Geometry: see drawing. Coordinates: mm, zero at the bounding-box minimum. Give positions to 0.01 mm unless a question says otherwise; leave off trailing zeros. Order: outer loops, then holes, each group sorted by start corner. A loop starts at its lowest first (then second) coordinate and runs counter-clockwise, first axis right, second up. Notation, with made-up numbers: (89.5, 10) -> (111.5, 10) arc R25 ccw to (111.5, 40) -> close; hole circle Ø5 at (79, 44). An arc over 180 degrees is marked (long way). One line per item, written item: value. Start each with the question number.
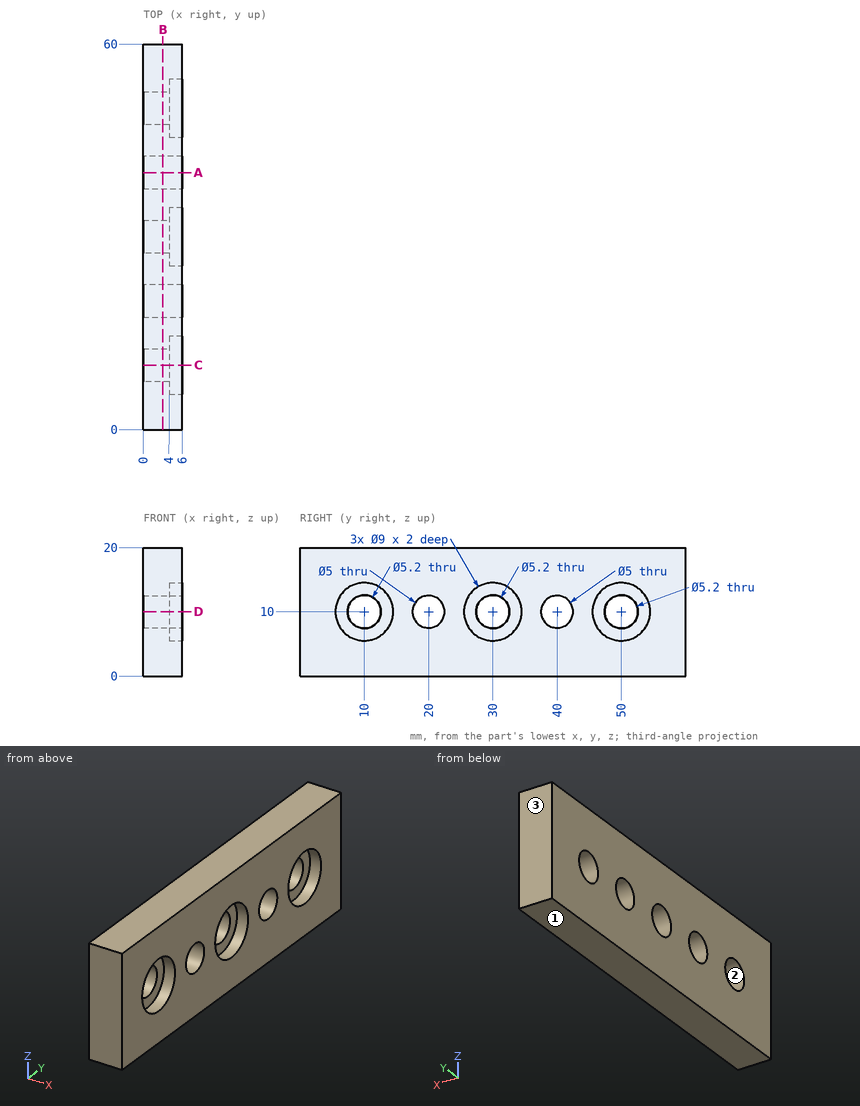
1. Pin query (flat end, axial travel): P1, Ø7, axis at y = 10, z = 10, coming from the +X side. Return the tip coordinate at first contact, or that it passes through.
2. Cut plane A-A, the plane y = 40. Return loops of the section in (x, z), then the cut area to 3 significant figures.
3. Draft query along Z for the marked faces 1, 2 and 3. Return one class per face: pulls with the +Z half, pulls with the -Z half, needs draft (parallel to the pull), parting line crosses it, or undercut.
4. Cut plane D-D, the plane z = 10. State how many separate pieces and enclosed holes the cut face has, then the cut area to 3 significant figures.
5. Cut plane B-B, the plane x = 3. Return loops of the section in (y, z).
6. Material intervals for L1, parallel to Z at x = 1.4, y = 10; L2, parallel to Z at x = 5.2, y = 50; L3, parallel to Y at x = 2, z = 12.25, sorted ascending. Write a range as [from, to].
7. Cut plane C-C, the plane y = 10. Return loops of the section in (x, z).
Answers follow:
1. P1: stops at x = 4
2. outline: (0, 0) -> (6, 0) -> (6, 7.5) -> (0, 7.5) -> close; (0, 12.5) -> (6, 12.5) -> (6, 20) -> (0, 20) -> close
2. area: 90.0 mm²
3. face 1: pulls with the -Z half
3. face 2: undercut
3. face 3: needs draft
4. separate pieces: 6
4. enclosed holes: 0
4. area: 184 mm²
5. outline: (0, 0) -> (60, 0) -> (60, 20) -> (0, 20) -> close; hole circle Ø5.2 at (10, 10); hole circle Ø5 at (20, 10); hole circle Ø5.2 at (30, 10); hole circle Ø5 at (40, 10); hole circle Ø5.2 at (50, 10)
6. L1: z = [0, 7.4], [12.6, 20]
6. L2: z = [0, 5.5], [14.5, 20]
6. L3: y = [0, 8.7], [11.3, 18.91], [21.09, 28.7], [31.3, 38.91], [41.09, 48.7], [51.3, 60]
7. outline: (0, 0) -> (6, 0) -> (6, 5.5) -> (4, 5.5) -> (4, 7.4) -> (0, 7.4) -> close; (0, 12.6) -> (4, 12.6) -> (4, 14.5) -> (6, 14.5) -> (6, 20) -> (0, 20) -> close
